Here's how the part is built. I have some questions about the finished solid (model axes, mm). A direction names the side the tool comes from. Coordinates: 2 decimals unless noted, no trailing zeros. Write each loop counter-clockwise with the first axis right and the second up, starting at its lowest first coordinate (ties: lowest second). Pieces come first, ordered by that corner, then holes. Notation, with made-up numbers: M 73.25,76.25 L 99.25,76.25 A8 cw 99.25,81.25 Z; hole C -19,23.25 d5. An arc over 180 degrees is marked long. Use one line per item in the form item = value. Start each with the question number.
1. Please list where these lines run through material, in increasing order: line 1 along X through (y, z) = (-20.3, 42.5); line 2 along X through (y, z) = (-19, 6); line 3 along Y through (x, z) = (-21.65, 24.5). Write a range as [from, to].
2. I want a section at B-B, the plane x = -6. List the corners of the cut face in (y, z) for me, plus the area to 3 significant figures.
3. On a 3-axis mill with a long thin cutter (end or side, diameter ignored), from which of +Z, -Z, +X, -X, +Y, -Y can I reach the whole of each face in a straight line? I mean faces 1 (the face through (-19.564, -0.1, 18.7)), 2 (the face through (33.745, -20.247, 43.458)). Say none if no direction works.
4. I want a section at D-D, the plane y = -0.5. List the corners of the cut face in (x, z) for me.
5. I want a section at C-C, the plane z = 6.5. List the corners of the cut face in (x, y) for me, plus the area to 3 significant figures.
6. I'm going to push flat-ended pins straight in: pin 1 Ø3 at (y, z) = (23, 11) entering from +X; pin 2 Ø8 at (x, y) = (-5.5, -15) entering from +Z; pin 3 Ø8 at (x, z) = (31.44, 6.5) entering from +Y. Where does each tip first touch, or does it pass through?
7. I want a section at A-A, the plane z = 24.5. List the corners of the cut face in (x, y) for me, plus the area to 3 significant figures.
8. Thinking about a two-plate mould opening in X: for faces 3 (the face through (11, -21.768, 24)), 4 (the face through (33.745, -20.247, 7.458)), 5 (the face through (-5.11, -20.25, 44.94)), 6 (the face through (46.436, -20, 24)), which applies, released by +X, released by -X, zero draft, split by the parting line, or undercut?
from build123d import *

# Parameters (mm, degrees)
EXTRUDE_1_DEPTH     = 49
SKETCH_2_R          = 2.5
CUT_EXTRUDE_1_DEPTH = 49
SKETCH_3_R          = 8
CUT_EXTRUDE_2_DEPTH = 49


with BuildPart() as part:
    # 草图1 → 凸台-拉伸1 (new body)
    with BuildSketch(Plane.XY):
        Polygon((-22.564432673, 30.231958763), (-22.564432673, -21.768041237), (46.435567327, -21.768041237), (46.435567327, -18.768041237), (-19.564432673, -18.768041237), (-19.564432673, 30.231958763), align=None)
    extrude(amount=EXTRUDE_1_DEPTH)

    # 草图2 → 切除-拉伸1 (cut)
    with BuildSketch(Plane(origin=(0, -18.768041237, 0), x_dir=(1, 0, 0), z_dir=(0, 1, 0))):
        with Locations((-4.564432673, -6.5)):
            Circle(SKETCH_2_R)
        with Locations((31.435567327, -6.5)):
            Circle(SKETCH_2_R)
        with Locations((-4.564432673, -42.5)):
            Circle(SKETCH_2_R)
        with Locations((31.435567327, -42.5)):
            Circle(SKETCH_2_R)
    extrude(amount=-CUT_EXTRUDE_1_DEPTH, mode=Mode.SUBTRACT)

    # 草图3 → 切除-拉伸2 (cut)
    with BuildSketch(Plane.ZY.offset(22.564432673)):
        with Locations((24.5, 5.731958763)):
            Circle(SKETCH_3_R)
    extrude(amount=-CUT_EXTRUDE_2_DEPTH, mode=Mode.SUBTRACT)


solid = part.part
Answer list:
q1.line_1 = [-22.56, -7.06], [-2.06, 28.94], [33.94, 46.44]
q1.line_2 = [-22.56, -7.01], [-2.11, 28.99], [33.89, 46.44]
q1.line_3 = [-21.77, -2.27], [13.73, 30.23]
q2.outline = M -21.77,0 L -18.77,0 L -18.77,4.45 L -21.77,4.45 Z; M -21.77,8.55 L -18.77,8.55 L -18.77,40.45 L -21.77,40.45 Z; M -21.77,44.55 L -18.77,44.55 L -18.77,49 L -21.77,49 Z
q2.area = 122 mm²
q3.face_1 = +Z, -Z, +X, +Y
q3.face_2 = +Y, -Y
q4.outline = M -22.56,0 L -19.56,0 L -19.56,19.48 L -22.56,19.48 Z; M -22.56,29.52 L -19.56,29.52 L -19.56,49 L -22.56,49 Z
q5.outline = M -22.56,-21.77 L -7.06,-21.77 L -7.06,-18.77 L -19.56,-18.77 L -19.56,30.23 L -22.56,30.23 Z; M -2.06,-21.77 L 28.94,-21.77 L 28.94,-18.77 L -2.06,-18.77 Z; M 33.94,-21.77 L 46.44,-21.77 L 46.44,-18.77 L 33.94,-18.77 Z
q5.area = 324 mm²
q6.pin_1 = -19.56
q6.pin_2 = 49
q6.pin_3 = -18.77
q7.outline = M -22.56,-21.77 L 46.44,-21.77 L 46.44,-18.77 L -19.56,-18.77 L -19.56,-2.27 L -22.56,-2.27 Z; M -22.56,13.73 L -19.56,13.73 L -19.56,30.23 L -22.56,30.23 Z
q7.area = 306 mm²
q8.face_3 = zero draft
q8.face_4 = undercut
q8.face_5 = undercut
q8.face_6 = released by +X
